Build history of the part. All positions in model axes, mm. Give positions to 0.01 mm unless a question says otherwise; leave off trailing zeros. Write each loop counter-clockwise with the first axis right and the second up, starting at its lowest first coordinate (ties: lowest second). Pieces come first, ordered by that corner, then holes. Notation, with made-up numbers: (-34.75, -19.5) -> (-28.75, -19.5) arc R21 cw to (-28.75, -1.5) -> close; hole circle Ø11 at (41, -36). An arc over 180 degrees is marked (long way). Put each result on its own line as item: value.
from build123d import *

# Parameters (mm, degrees)
F0_W         = 127
F0_H         = 76.2
F0_R         = 6.8502620854
F0_R_2       = 6.35
F1_DEPTH     = 50.8
F2_R         = 6.7087058048
F3_DEPTH     = 127
F4_T1_DEPTH  = 6.4524666085
F4_T3_DEPTH  = 6.4524666085
F4_T5_DEPTH  = 6.4524666085
F4_T7_DEPTH  = 6.4524666085
F4_T9_DEPTH  = 6.4524666085
F4_T11_DEPTH = 6.4524666085
F4_T13_DEPTH = 6.4524666085
F4_T15_DEPTH = 6.4524666085
F4_T17_DEPTH = 102.3282991577
F4_T19_DEPTH = 153.1282991577
F4_T21_DEPTH = 76.9282991577
F5_T1_DEPTH  = 15.2572709249
F5_T3_DEPTH  = 76.5610244843


# Not quite as in the source:
# - a fillet or chamfer that OpenCascade refuses, or shapes differently, is made with other operations: its cross-section is extruded or revolved along the edge and cut away or added


with BuildPart() as f1:
    # F0 (on Front) → F1 (new body)
    with BuildSketch(Plane.XZ):
        with Locations((-63.5, 38.1)):
            Rectangle(F0_W, F0_H)
        with Locations((-110.5553433299, 66.1175847054)):
            Circle(F0_R, mode=Mode.SUBTRACT)
        with Locations((-19.05, 50.8)):
            Circle(F0_R_2, mode=Mode.SUBTRACT)
    extrude(amount=F1_DEPTH)

    # F2 (on face) → F3 (cut)
    with BuildSketch(Plane.XZ.offset(50.8)):
        with Locations((-109.2690080404, 36.7891639471)):
            Circle(F2_R)
    extrude(amount=-F3_DEPTH, mode=Mode.SUBTRACT)

    # F4: chamfer of 5.08 on 12 edges, made by hand

    # F4_s2 → F4_t1 (cut)
    with BuildSketch(Plane(origin=(-81.28, -81.28, 81.28), x_dir=(0.7071067812, -0.7071067812, 0), z_dir=(-0.5773502692, -0.5773502692, 0.5773502692))):
        Polygon((-53.8815367264, -6.2217039467), (-57.4736391748, -12.4434078933), (-50.289434278, -12.4434078933), align=None)
    extrude(amount=F4_T1_DEPTH, mode=Mode.SUBTRACT)

    # F4_s4 → F4_t3 (cut)
    with BuildSketch(Plane(origin=(-55.88, -55.88, -55.88), x_dir=(0.7071067812, -0.7071067812, 0), z_dir=(-0.5773502692, -0.5773502692, -0.5773502692))):
        Polygon((-57.4736391748, 74.66044736), (-50.289434278, 74.66044736), (-53.8815367264, 68.4387434134), align=None)
    extrude(amount=F4_T3_DEPTH, mode=Mode.SUBTRACT)

    # F4_s6 → F4_t5 (cut)
    with BuildSketch(Plane(origin=(38.9466666667, -38.9466666667, 38.9466666667), x_dir=(0.7071067812, 0.7071067812, 0), z_dir=(0.5773502692, -0.5773502692, 0.5773502692))):
        Polygon((-35.9210244843, 45.6258289422), (-32.3289220358, 39.4041249956), (-39.5131269327, 39.4041249956), align=None)
    extrude(amount=F4_T5_DEPTH, mode=Mode.SUBTRACT)

    # F4_s8 → F4_t7 (cut)
    with BuildSketch(Plane(origin=(-64.3466666667, 64.3466666667, 64.3466666667), x_dir=(-0.7071067812, -0.7071067812, 0), z_dir=(-0.5773502692, 0.5773502692, 0.5773502692))):
        Polygon((89.8025612107, 14.5173092089), (93.3946636591, 8.2956052622), (86.2104587623, 8.2956052622), align=None)
    extrude(amount=F4_T7_DEPTH, mode=Mode.SUBTRACT)

    # F4_s10 → F4_t9 (cut)
    with BuildSketch(Plane(origin=(-38.9466666667, 38.9466666667, -38.9466666667), x_dir=(-0.7071067812, -0.7071067812, 0), z_dir=(-0.5773502692, 0.5773502692, -0.5773502692))):
        Polygon((93.3946636591, 53.9214342045), (86.2104587623, 53.9214342045), (89.8025612107, 47.6997302578), align=None)
    extrude(amount=F4_T9_DEPTH, mode=Mode.SUBTRACT)

    # F4_s12 → F4_t11 (cut)
    with BuildSketch(Plane(origin=(22.0133333333, 22.0133333333, 22.0133333333), x_dir=(-0.7071067812, 0.7071067812, 0), z_dir=(0.5773502692, 0.5773502692, 0.5773502692))):
        Polygon((0, 66.3648420978), (-3.5921024484, 60.1431381511), (3.5921024484, 60.1431381511), align=None)
    extrude(amount=F4_T11_DEPTH, mode=Mode.SUBTRACT)

    # F4_s14 → F4_t13 (cut)
    with BuildSketch(Plane(origin=(-3.3866666667, -3.3866666667, 3.3866666667), x_dir=(-0.7071067812, 0.7071067812, 0), z_dir=(0.5773502692, 0.5773502692, -0.5773502692))):
        Polygon((-3.5921024484, 2.0739013156), (3.5921024484, 2.0739013156), (0, -4.1478026311), align=None)
    extrude(amount=F4_T13_DEPTH, mode=Mode.SUBTRACT)

    # F4_s16 → F4_t15 (cut)
    with BuildSketch(Plane(origin=(13.5466666667, -13.5466666667, -13.5466666667), x_dir=(0.7071067812, 0.7071067812, 0), z_dir=(0.5773502692, -0.5773502692, -0.5773502692))):
        Polygon((-32.3289220358, 22.8129144711), (-39.5131269327, 22.8129144711), (-35.9210244843, 16.5912105245), align=None)
    extrude(amount=F4_T15_DEPTH, mode=Mode.SUBTRACT)

    # F4_s18 → F4_t17 (cut)
    with BuildSketch(Plane.XY.offset(-13.0641495789)):
        Polygon((-127, -45.72), (-121.92, -50.8), (-127, -50.8), align=None)
        Polygon((-127, -5.08), (-121.92, 0), (-127, 0), align=None)
        Polygon((0, -45.72), (-5.08, -50.8), (0, -50.8), align=None)
        Polygon((0, -5.08), (-5.08, 0), (0, 0), align=None)
    extrude(amount=F4_T17_DEPTH, mode=Mode.SUBTRACT)

    # F4_s20 → F4_t19 (cut)
    with BuildSketch(Plane.YZ.offset(-140.0641495789)):
        Polygon((-45.72, 76.2), (-50.8, 71.12), (-50.8, 76.2), align=None)
        Polygon((-5.08, 76.2), (0, 71.12), (0, 76.2), align=None)
        Polygon((0, 5.08), (-5.08, 0), (0, 0), align=None)
        Polygon((-50.8, 5.08), (-45.72, 0), (-50.8, 0), align=None)
    extrude(amount=F4_T19_DEPTH, mode=Mode.SUBTRACT)

    # F4_s22 → F4_t21 (cut)
    with BuildSketch(Plane.XZ.offset(-13.0641495789)):
        Polygon((-127, 5.08), (-121.92, 0), (-127, 0), align=None)
        Polygon((-121.92, 76.2), (-127, 71.12), (-127, 76.2), align=None)
        Polygon((0, 5.08), (-5.08, 0), (0, 0), align=None)
        Polygon((-5.08, 76.2), (0, 71.12), (0, 76.2), align=None)
    extrude(amount=F4_T21_DEPTH, mode=Mode.SUBTRACT)

    # F5: fillet of radius 5.08 on 4 edges, made by hand

    # F5_s2 → F5_t1 (cut)
    with BuildSketch(Plane(origin=(-43.4942598667, 43.4942598667, 0), x_dir=(0, 0, 1), z_dir=(0.7071067812, -0.7071067812, 0))):
        with BuildLine():
            ThreePointArc((6.6946132056, 122.1314832465), (5.1558535372, 121.892827965), (3.7616738381, 121.1992858777))
            Line((3.7616738381, 121.1992858777), (5.08, 122.1314832465))
            Line((5.08, 122.1314832465), (6.6946132056, 122.1314832465))
        make_face()
        with BuildLine():
            ThreePointArc((72.4383261619, 121.1992858777), (71.0441464628, 121.892827965), (69.5053867944, 122.1314832465))
            Line((69.5053867944, 122.1314832465), (71.12, 122.1314832465))
            Line((71.12, 122.1314832465), (72.4383261619, 121.1992858777))
        make_face()
    extrude(amount=F5_T1_DEPTH, mode=Mode.SUBTRACT)

    # F5_s4 → F5_t3 (cut)
    with BuildSketch(Plane.XY.offset(-0.1805122422)):
        with BuildLine():
            ThreePointArc((-119.8157951031, -50.8), (-121.7598269396, -50.4133080252), (-123.4078975516, -49.3121024484))
            Line((-123.4078975516, -49.3121024484), (-121.92, -50.8))
            Line((-121.92, -50.8), (-119.8157951031, -50.8))
        make_face()
        with BuildLine():
            ThreePointArc((-127, -43.6157951031), (-126.6133080252, -45.5598269396), (-125.5121024484, -47.2078975516))
            Line((-125.5121024484, -47.2078975516), (-127, -45.72))
            Line((-127, -45.72), (-127, -43.6157951031))
        make_face()
    extrude(amount=F5_T3_DEPTH, mode=Mode.SUBTRACT)


solid = f1.part
1) Pull direction X, two halves, no side cores. Call faces 1 (the cylindrical face through (-124.3, -48.1, 5.2)), 2 (the cylindrical face through (-19.877, -25.044, 57.096)), 3 (the flat face through (-63, -50.8, 39)): released by +X, released by -X, zero draft, split by the parting line, or undercut.
Filled sheet:
face 1: released by -X
face 2: undercut
face 3: zero draft
2) Slice it at B-B (x = -19.05). Write the cut outline in (y, z), plus the area to 3 significant figures.
Filled sheet:
outline: (-50.8, 5.08) -> (-45.72, 0) -> (-5.08, 0) -> (0, 5.08) -> (0, 44.45) -> (-50.8, 44.45) -> close; (-50.8, 57.15) -> (0, 57.15) -> (0, 71.12) -> (-5.08, 76.2) -> (-45.72, 76.2) -> (-50.8, 71.12) -> close
area: 3,170 mm2
3) Slice it at A-A (z = 50.8). Write the cut outline in (x, y), plus the area to 3 significant figures.
Filled sheet:
outline: (-127, -43.62) arc R5.08 ccw to (-125.51, -47.21) -> (-123.41, -49.31) arc R5.08 ccw to (-119.82, -50.8) -> (-25.4, -50.8) -> (-25.4, 0) -> (-121.92, 0) -> (-127, -5.08) -> close; (-12.7, -50.8) -> (-5.08, -50.8) -> (0, -45.72) -> (0, -5.08) -> (-5.08, 0) -> (-12.7, 0) -> close
area: 5,750 mm2
4) Slice it at D-D (z = 39). Write the cut outline in (x, y), plus the area to 3 significant figures.
Filled sheet:
outline: (-127, -43.62) arc R5.08 ccw to (-125.51, -47.21) -> (-123.41, -49.31) arc R5.08 ccw to (-119.82, -50.8) -> (-115.6, -50.8) -> (-115.6, 0) -> (-121.92, 0) -> (-127, -5.08) -> close; (-102.94, -50.8) -> (-5.08, -50.8) -> (0, -45.72) -> (0, -5.08) -> (-5.08, 0) -> (-102.94, 0) -> close
area: 5,760 mm2
5) Wall check: L1, parallel to Z at x = -19, y = -11; L2, parallel to X at y = -31, z = 66; L3, parallel to Z at x = -113, y = -15.5. Give the ranges that are in metal, low to high.
Filled sheet:
L1: 0 to 44.45, 57.15 to 76.2
L2: -127 to -117.4, -103.71 to 0
L3: 0 to 31.21, 42.36 to 59.72, 72.52 to 76.2
6) Slice it at C-C (y = -30). Write the cut outline in (x, z), plus the area to 3 significant figures.
Filled sheet:
outline: (-127, 5.08) -> (-121.92, 0) -> (-5.08, 0) -> (0, 5.08) -> (0, 71.12) -> (-5.08, 76.2) -> (-121.92, 76.2) -> (-127, 71.12) -> close; hole circle Ø13.7 at (-110.56, 66.12); hole circle Ø13.42 at (-109.27, 36.79); hole circle Ø12.7 at (-19.05, 50.8)
area: 9,210 mm2
